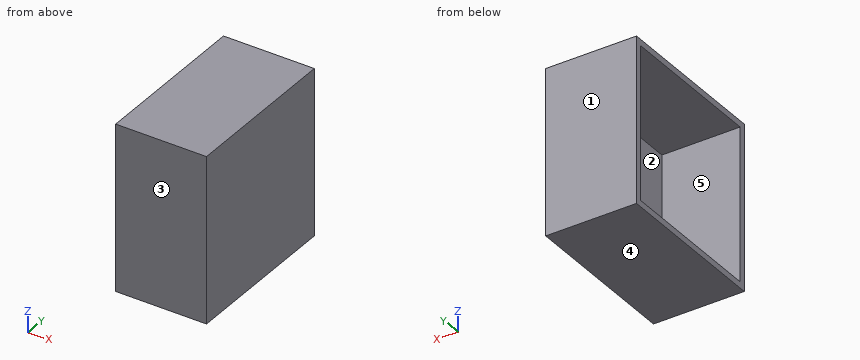
Autodesk Inventor part; units mm, degrees
ref_plane "YZ Plane" through (0, 0, 0) normal (1, 0, 0) x (0, 1, 0)
ref_plane "XZ Plane" through (0, 0, 0) normal (0, 1, 0) x (-1, 0, 0)
ref_plane "XY Plane" through (0, 0, 0) normal (0, 0, 1) x (1, 0, 0)
sketch "Sketch1" plane through (0, 0, 0) normal (1, 0, 0) x (0, 1, 0)
  line L0 (-12, 12.25) -> (12, 12.25)
  line L1 (12, 12.25) -> (12, -12.25)
  line L2 (12, -12.25) -> (-12, -12.25)
  line L3 (-12, -12.25) -> (-12, 12.25)
  line L4 (-12, 12.25) -> (12, -12.25) construction
  line L5 (12, 12.25) -> (-12, -12.25) construction
  line L6 (-13, -13.25) -> (13, -13.25)
  line L7 (13, -13.25) -> (13, 13.25)
  line L8 (13, 13.25) -> (-13, 13.25)
  line L9 (-13, 13.25) -> (-13, -13.25)
  line L10 (-13, -13.25) -> (13, 13.25) construction
  line L11 (13, -13.25) -> (-13, 13.25) construction
  point P0 (0, 0)
  dimension "d0" = 24
  dimension "d1" = 24.5
  dimension "d2" = 26
  dimension "d3" = 26.5
extrude "Extrusion1" add sketch "Sketch1" along normal blind 14.5
sketch "Sketch2" plane through (0, 13, 13.25) normal (0, 1, 0) x (1, 0, 0)
  line L0 (0, 26.5) -> (14.5, 26.5)
  line L1 (0, 0) -> (14.5, 0)
  line L2 (14.5, 26.5) -> (12.5, 26.5)
  line L3 (12.5, 26.5) -> (12.5, 0)
  line L4 (12.5, 0) -> (14.5, 0)
  line L5 (14.5, 0) -> (14.5, 26.5)
  point P0 (0, 13.25)
  dimension "d6" = 2
extrude "Extrusion2" add sketch "Sketch2" against normal blind 26
sketch "Sketch3" plane through (0, 0, 0) normal (-1, 0, 0) x (0, 0, 1)
  point P0 (0, 0)
properties part number "servoHolderBase"
Source: CAD feature listing. Evaluate the final solid. Frame: model axes, mm. Face numbers are marked on the shaded views. A direction names the side the tool comes from. Coordinates: 2 decimals unless noted, no trailing zeros. Loops run counter-clockwise (first coordinate to the right, second up) from the corner with the lowest first, then second, coordinate; pieces in that order, holes last. Notation, with made-up numbers: M 2.25,87.5 L 44.25,87.5 A23 cw 44.25,105.5 Z; hole C 82,5.25 d3. An arc over 180 degrees is marked long. Put each result on its own line as item: value. Start each with the question number.
1) Cut plane C-C on z = -1. Return the cut outline in (x, y).
2) Ray query, L1, parallel to Y at x = 11.75, z = 4.5; L2, parallel to Z at x = 8.25, y = -7; L3, parallel to X at y = 10.5, z = 2.5. Return the intervals inside material, ascending. Write a range as from..to.
3) Contact query for a flat-ended pin moving along its axis: pin 1 Ø1 at (y, z) = (4, 5) entering from -X. Output: stop coordinate, or through.
4) Reachability of the marked faces 1 and 2 from +Z, -Z, +X, -X, +Y, -Y: full face, straight path, thin tool, end or side. Return the list, or none.
5) Cut plane B-B on y = -7.5. Return the cut outline in (x, z), then the cut area to 3 significant figures.
6) Pull-direction query (Y, two-part tool) for the marked faces 3, 4 and 5; classes: pulls with the +Y half, pulls with the -Y half, needs draft (parallel to the pull), parting line crosses it, or undercut.
7) Cut plane A-A on x = 9.25. Return the cut outline in (y, z), then the cut area to 3 significant figures.
The answers:
1. outline: M 0,-13 L 14.5,-13 L 14.5,13 L 0,13 L 0,12 L 12.5,12 L 12.5,-12 L 0,-12 Z
2. L1: y = -13..-12, 12..13
2. L2: z = -13.25..-12.25, 12.25..13.25
2. L3: x = 12.5..14.5
3. pin 1: stops at x = 12.5
4. face 1: +Z, -Z, +X, -X, +Y
4. face 2: -X
5. outline: M 0,-13.25 L 14.5,-13.25 L 14.5,13.25 L 0,13.25 L 0,12.25 L 12.5,12.25 L 12.5,-12.25 L 0,-12.25 Z
5. area: 78.0 mm²
6. face 3: pulls with the -Y half
6. face 4: needs draft
6. face 5: undercut
7. outline: M -13,-13.25 L 13,-13.25 L 13,13.25 L -13,13.25 Z; hole M -12,-12.25 L 12,-12.25 L 12,12.25 L -12,12.25 Z
7. area: 101 mm²
